Geometry check sheet. Reference: drawing and pictorial views, mm from the part's lowest x, y, z. A direction names the side the tool comes from. Round coordinates to 2 decimals unless told otherwise and drop trailing zeros. Loops run counter-clockwise (first coordinate to the right, second up) from the corner with the lowest first, then second, coordinate; pieces in that order, holes last. Notation, with made-up numbers: (14, 12) - (42, 12) arc R21 ccw to (42, 41) - close; hole circle Ø11 at (80.25, 41). An arc over 180 degrees is marked (long way). Answer as CSV lines item,"result". Start each with the question number.
1) Thickness scan on line 1 along Y through (x, z) = (30, 4); line 2 along Y through (x, z) = (30, 14); line 3 along Z through (x, y) = (13.5, 28). Record the ranges inside material, lowest first.
2) Cross-section at A-A on x = 30. Record the boundary of the cut face in (y, z).
3) Cross-section at B-B on z = 6. Record the boundary of the cut face in (x, y).
4) Draft check along Y on the marked faces 1, 2 and 3. Enter one of: released by +Y, released by -Y, zero draft, split by the parting line, or undercut.
5) Cross-section at C-C on z = 31.5. State how many separate pieces and enclosed holes the cut face has, and give its area (3 significant figures).
6) Depth check by flat-ended pin: P1, Ø5, axis at y = 15, z = 17, coming from the +X side; P2, Ø10, axis at x = 29.5, z = 17, coming from the -Y side; P3, Ø2.5, axis at y = 73, z = 16, coming from the -X side. Enter the tip coordinate at first touch or a pass-through.
7) Access from +Z, -Z, +X, -X, +Y, -Y to the whole of each face (thin tool, end or side, straight path). Record for the marked faces 4, 5, 6 and 7.
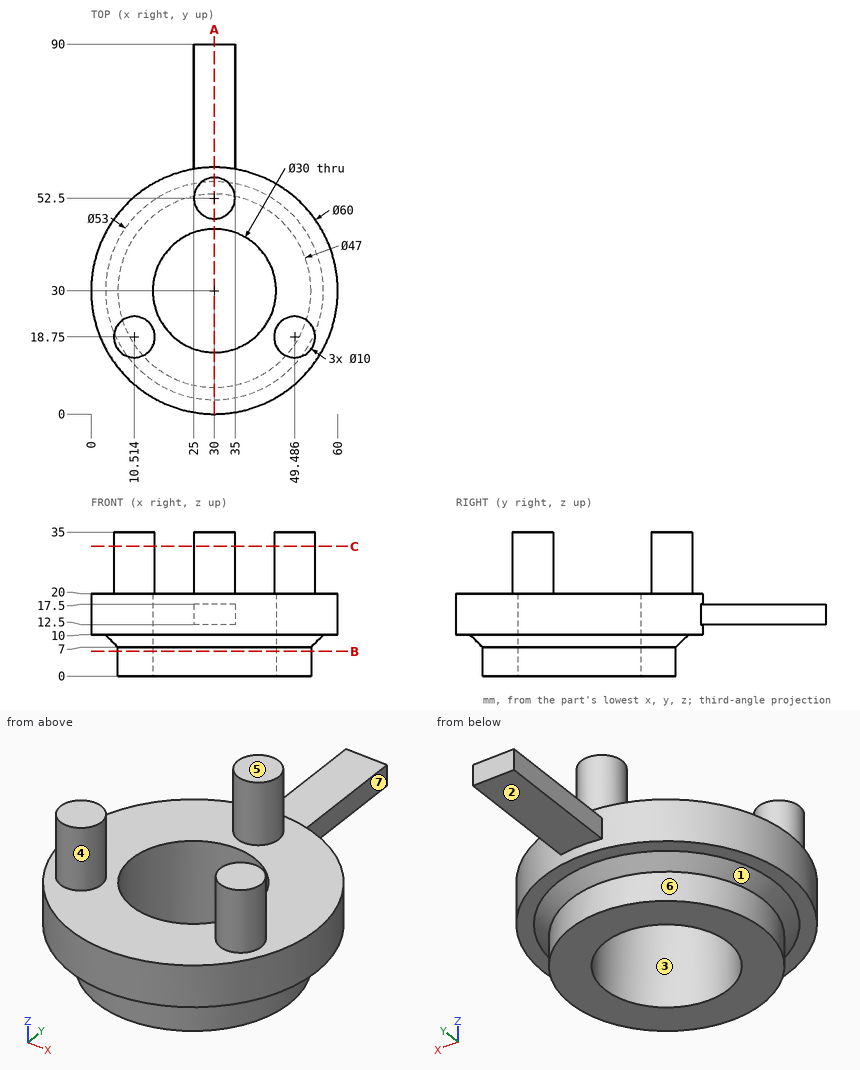
Answer block:
1,line 1,"y = 6.5 to 15, 45 to 53.5"
1,line 2,"y = 0 to 15, 45 to 90"
1,line 3,"z = 0 to 20"
2,outline,"(0, 10) - (3.5, 10) - (6.5, 7) - (6.5, 0) - (15, 0) - (15, 20) - (0, 20) - close; (45, 0) - (53.5, 0) - (53.5, 7) - (56.5, 10) - (60, 10) - (60, 12.5) - (90, 12.5) - (90, 17.5) - (60, 17.5) - (60, 20) - (57.5, 20) - (57.5, 35) - (47.5, 35) - (47.5, 20) - (45, 20) - close"
3,outline,"circle Ø47 at (30, 30); hole circle Ø30 at (30, 30)"
4,face 1,"split by the parting line"
4,face 2,"zero draft"
4,face 3,"undercut"
5,separate pieces,"3"
5,enclosed holes,"0"
5,area,"236 mm^2"
6,P1,"stops at x = 57.27"
6,P2,"stops at y = 0"
6,P3,"stops at x = 25"
7,face 4,"+Z"
7,face 5,"+Z, +X, -X, +Y, -Y"
7,face 6,"-Z"
7,face 7,"+Z, -Z, +X, +Y"
